Solid Edge part; units mm, degrees
sketch "Sketch1" plane through (0, 0, 0) normal (0, 0, 1) x (1, 0, 0)
  circle A0 centre (0, 0) radius 4.5
extrude "Protrusion1" add sketch "Sketch1" against normal blind 10
sketch "Sketch2" plane through (0, 0, 0) normal (0, 0, 1) x (1, 0, 0)
  line L0 (-11, -4.5) -> (11, -4.5)
  line L1 (11, -4.5) -> (11, 4.5)
  line L2 (11, 4.5) -> (-11, 4.5)
  line L3 (-11, 4.5) -> (-11, -4.5)
  dimension "D1" = 11
  dimension "D2" = 11
extrude "Extrusionsausprägung_2" add sketch "Sketch2" along normal blind 3
sketch "Sketch3" plane through (0, 0, 3) normal (0, 0, 1) x (1, 0, 0)
  circle A0 centre (-9, 0) radius 1.6
  circle A1 centre (9, 0) radius 1.6
  dimension "D1" = 9
extrude "Cutout1" cut sketch "Sketch3" against normal through all
sketch "Sketch4" plane through (0, 0, -10) normal (0, 0, -1) x (1, 0, 0)
  line L0 (-10, -4) -> (10, -4)
  line L1 (10, -4) -> (10, 4)
  line L2 (10, 4) -> (-10, 4)
  line L3 (-10, 4) -> (-10, -4)
  dimension "D1" = 10
  dimension "D2" = 10
extrude "Extrusionsausprägung_3" add sketch "Sketch4" along normal blind 30
sketch "Sketch5" plane through (0, -4, -25) normal (0, -1, 0) x (1, 0, 0)
  line L0 (-10, -15) -> (-0.5, -21)
  line L1 (-0.5, -21) -> (-0.5, -25)
  line L2 (-0.5, -25) -> (0.5, -25)
  line L3 (0.5, -25) -> (0.5, -21)
  line L4 (0.5, -21) -> (10, -15)
  line L5 (10, -15) -> (-10, -15)
  dimension "D1" = 0.5
  dimension "D2" = 0.5
extrude "Protrusion2" add sketch "Sketch5" against normal up to vertex (8 mm away)
sketch "Sketch6" plane through (10, 0, -25) normal (1, 0, 0) x (0, 1, 0)
  line L0 (-4, -15) -> (-0.5, -21)
  line L1 (-0.5, -21) -> (-0.5, -25)
  line L2 (-0.5, -25) -> (0.5, -25)
  line L3 (0.5, -25) -> (0.5, -21)
  line L4 (0.5, -21) -> (4, -15)
  dimension "D1" = 0.5
extrude "Cutout2" cut sketch "Sketch6" against normal through all material side at (10, -2.2932, -43.0252)
properties part number "A7.E1"
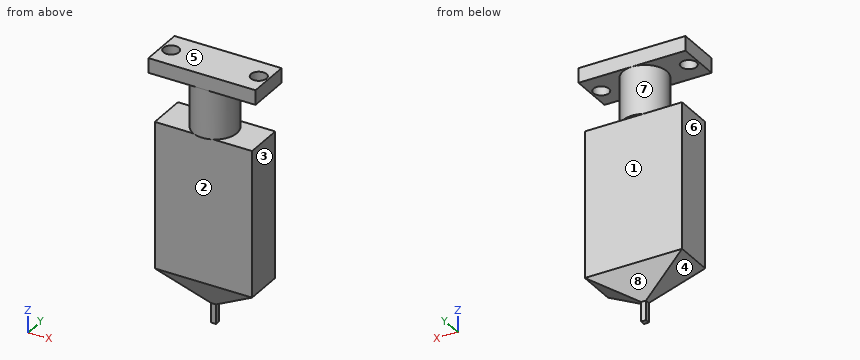
The listing builds one solid part. Answer for the finished solid, in the listing's coordinates (mm). Face numbers are marked on the shaded views. A direction names the side the tool comes from. Give positions to 0.01 mm unless a question says otherwise; leave off trailing zeros. Loops run counter-clockwise (first coordinate to the right, second up) from the corner with the lowest first, then second, coordinate; pieces in that order, holes last. Notation, with made-up numbers: M 26.5,43 L 69.5,43 A18 cw 69.5,73 Z; hole C 22.5,57.5 d10. An arc over 180 degrees is marked long. One line per item, written item: value.
Q1. Determine the mould class of the marked faces 6, 7 and 8 for opening direction X: +X half, -X half, draft (parallel to the pull), parting line (faces both ways), or undercut.
Working result:
face 6: -X half
face 7: parting line
face 8: draft
Q2. Find the intervals of material crossed by line 1 (Y direction, x = -9, z = 0.8); line 2 (Y direction, x = 6, z = -14.5); line 3 (Z direction, x = 5, y = -2), in increasing order. Write a range as from..to.
Working result:
line 1: y = -4.5..-1.6, 1.6..4.5
line 2: y = -4..4
line 3: z = -43.16..-10, 0..3
Q3. A cutting plane is placed at D-D on z = -30. Determine the outline of the cut face in (x, y), then the cut area to 3 significant figures.
Working result:
outline: M -10,-4 L 10,-4 L 10,4 L -10,4 Z
area: 160 mm^2
Q4. A cutting plane is placed at C-C on y = -2.25. Determine the outline of the cut face in (x, z), then the cut area to 3 significant figures.
Working result:
outline: M -11,0 L -3.9,0 L -3.9,-10 L -10,-10 L -10,-40 L -5.25,-43 L 5.25,-43 L 10,-40 L 10,-10 L 3.9,-10 L 3.9,0 L 11,0 L 11,3 L -11,3 Z
area: 790 mm^2
Q5. For the marked faces 1, 2, 3, 4 and 5, determine the directions among +Z, -Z, +X, -X, +Y, -Y from which every point of the face is accessible in a straight line to the end or side of a thin tool.
Working result:
face 1: -Z, +X, -X, +Y
face 2: -Z, +X, -X, -Y
face 3: -Z, +X, +Y, -Y
face 4: -Z, -X, +Y, -Y
face 5: +Z, +X, -X, +Y, -Y
Q6. A cutting plane is placed at B-B on x = -4. Determine the outline of the cut face in (y, z).
Working result:
outline: M -4.5,0 L -2.06,0 L -2.06,-10 L -4,-10 L -4,-40 L -1.79,-43.79 L 1.79,-43.79 L 4,-40 L 4,-10 L 2.06,-10 L 2.06,0 L 4.5,0 L 4.5,3 L -4.5,3 Z
Q7. A cutting plane is placed at A-A on x = 9. Determine the outline of the cut face in (y, z).
Working result:
outline: M -4.5,0 L -1.6,0 L -1.6,3 L -4.5,3 Z; M -4,-40 L -3.63,-40.63 L 3.63,-40.63 L 4,-40 L 4,-10 L -4,-10 Z; M 1.6,0 L 4.5,0 L 4.5,3 L 1.6,3 Z
Q8. Flat-ended cylindrical pins translate along their axes: P1, Ø3, axis at x = 3.5, z = -16, coming from the +Y side; P2, Ø0.8, axis at y = 0, z = -48.5, coming from the +X side; P3, Ø1, axis at x = 6, z = -18, coming from the -Y side. Find the tip coordinate at first contact, or state that the pin passes through.
Working result:
P1: stops at y = 4
P2: stops at x = 0.5
P3: stops at y = -4
